Geometry check sheet. Reference: drawing and pictorial views, mm from the part's lowest x, y, z. Round coordinates to 2 decimals unless told otherwise and drop trailing zeros. Write each loop counter-clockwise with the first axis right and the second up, starting at its lowest first coordinate (ties: lowest second). Pieces come first, ordered by that corner, then holes. Notation, with made-up numbers: M 71,20.5 L 104,20.5 A24 cw 104,53.5 Z; hole C -33,-1 d5. An arc over 180 degrees is marked long. Answer in a Markdown table with one row per item. Add a question column.
1. Sectioned sample at A-A on z = 5.5. Record the cut outline in (x, y).
2. Sectioned sample at D-D on y = 1.4. Record the cut outline in (x, z).
3. Sectioned sample at C-C on z = 21. Record the cut outline in (x, y).
4. Sectioned sample at B-B on x = 21. Record the cut outline in (y, z), plus the area to 3 significant figures.
5. Material ranges on probe 1 along X at (y, z) = (1.6, 5.5); probe 2 along X at (y, z) = (2.4, 5); probe 3 along X at (y, z) = (0.85, 21.5), recorded low to high.
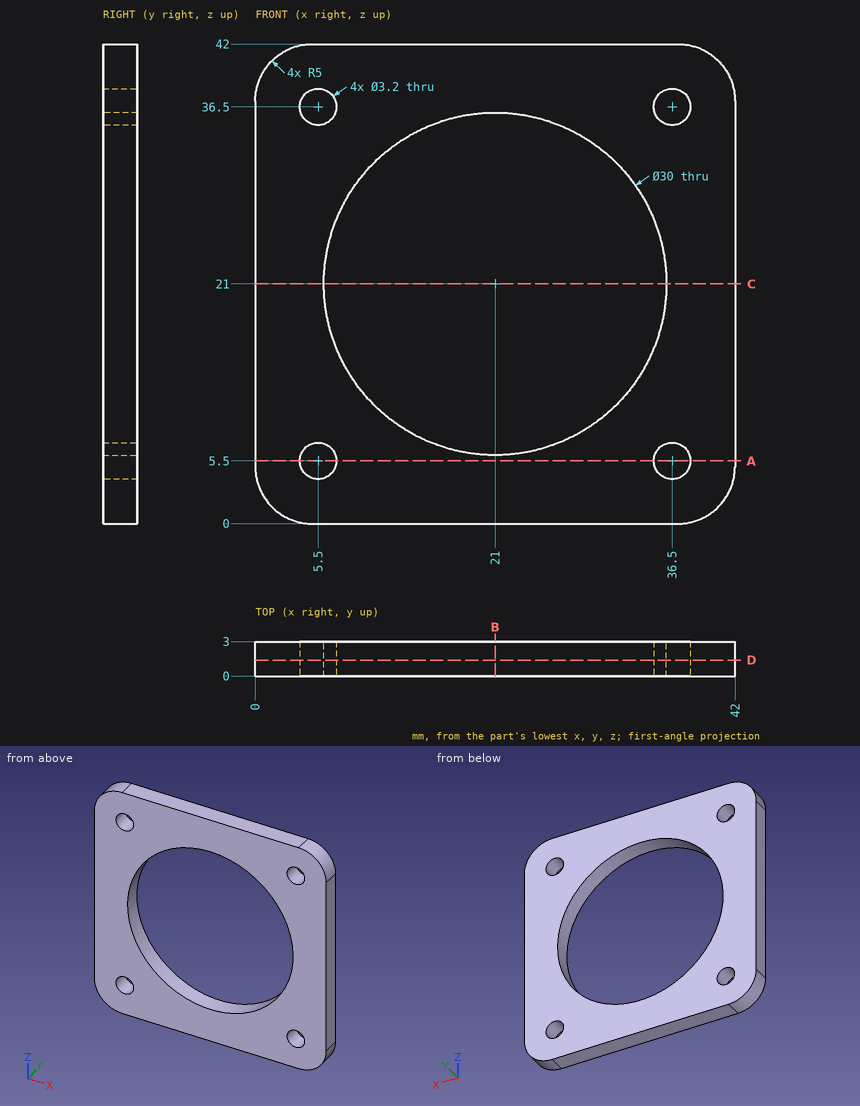
Geometry check:
| question | item | result |
|---|---|---|
| 1 | outline | M 0,0 L 3.9,0 L 3.9,3 L 0,3 Z; M 7.1,0 L 34.9,0 L 34.9,3 L 7.1,3 Z; M 38.1,0 L 42,0 L 42,3 L 38.1,3 Z |
| 2 | outline | M 0,5 A5 ccw 5,0 L 37,0 A5 ccw 42,5 L 42,37 A5 ccw 37,42 L 5,42 A5 ccw 0,37 Z; hole C 5.5,5.5 d3.2; hole C 5.5,36.5 d3.2; hole C 21,21 d30; hole C 36.5,5.5 d3.2; hole C 36.5,36.5 d3.2 |
| 3 | outline | M 0,0 L 6,0 L 6,3 L 0,3 Z; M 36,0 L 42,0 L 42,3 L 36,3 Z |
| 4 | outline | M 0,0 L 3,0 L 3,6 L 0,6 Z; M 0,36 L 3,36 L 3,42 L 0,42 Z |
| 4 | area | 36.0 mm2 |
| 5 | probe 1 | x = 0 to 3.9, 7.1 to 34.9, 38.1 to 42 |
| 5 | probe 2 | x = 0 to 3.98, 7.02 to 34.98, 38.02 to 42 |
| 5 | probe 3 | x = 0 to 6.01, 35.99 to 42 |
